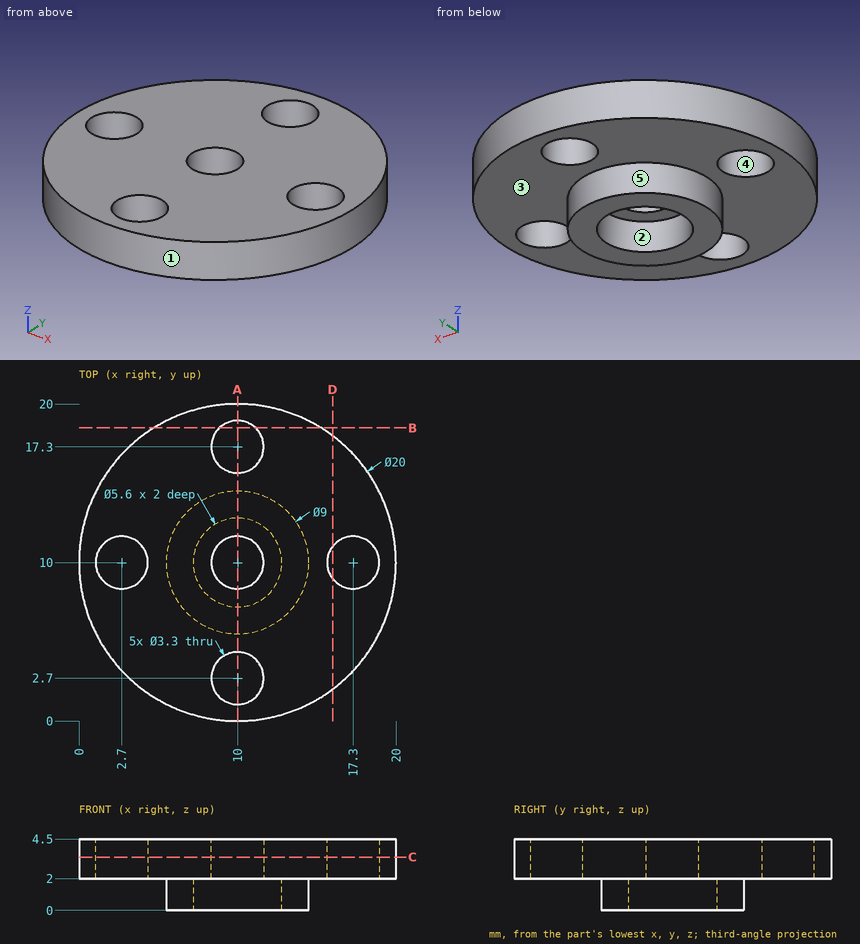
Here's the drawing with two shaded views (mm, measured from the low corner). I have some questions. A direction names the side the tool comes from. Give positions to 0.01 mm unless a question says otherwise; leave off trailing zeros. Order: outer loops, then holes, each group sorted by start corner. A loop starts at its lowest first (then second) coordinate and runs counter-clockwise, first axis right, second up. Notation, with made-up numbers: (4.5, -37) - (61.5, -37) arc R27 cw to (61.5, -1) - close; hole circle Ø9 at (58, 5). An arc over 180 degrees is marked (long way). Use a Markdown table: item, result. Add a question column.
Q1. On a 3-axis mill with a long thin cutter (end or side, diameter ignored), from which of +Z, -Z, +X, -X, +Y, -Y can I reach the whole of each face in a straight line? I mean the marked faces 4 and 5. Say none if no direction works.
Q2. If we section it at D-D on x = 16: Write out the boundary of the cut face in (y, z).
Q3. If we section it at B-B on y = 18.5: Write out the boundary of the cut face in (x, z).
Q4. If we section it at C-C on z = 3.35: Write out the boundary of the cut face in (x, y), plus the area to 3 significant figures.
Q5. If we section it at A-A on x = 10: Write out the boundary of the cut face in (y, z), plus the area to 4 significant figures.
Q6. Please list where these lines run through material, in increasing order: line 1 along Y through (x, z) = (10, 3.45); line 2 along Z through (x, y) = (7, 14.75); line 3 along X through (y, z) = (12, 1.35).
Q7. If we mould it in two halves opening along Y, with no side actions, what happens to the marked faces 1, 2 and 3? For each: released by +Y, released by -Y, zero draft, split by the parting line, or undercut.
Q8. I'm going to push flat-ended pins straight in: pin 1 (6 mm diameter, centred on x = 17.5, y = 9, fed in from -Z); pin 2 (2 mm diameter, centred on y = 13, z = 2, fed in from -X). Where does each tip first touch, or does it pass through?
Answers follow:
| question | item | result |
|---|---|---|
| 1 | face 4 | +Z, -Z |
| 1 | face 5 | -Z |
| 2 | outline | (2, 2) - (8.98, 2) - (8.98, 4.5) - (2, 4.5) - close; (11.02, 2) - (18, 2) - (18, 4.5) - (11.02, 4.5) - close |
| 3 | outline | (4.73, 2) - (8.87, 2) - (8.87, 4.5) - (4.73, 4.5) - close; (11.13, 2) - (15.27, 2) - (15.27, 4.5) - (11.13, 4.5) - close |
| 4 | outline | circle Ø20 at (10, 10); hole circle Ø3.3 at (2.7, 10); hole circle Ø3.3 at (10, 2.7); hole circle Ø3.3 at (10, 10); hole circle Ø3.3 at (10, 17.3); hole circle Ø3.3 at (17.3, 10) |
| 4 | area | 271 mm^2 |
| 5 | outline | (0, 2) - (1.05, 2) - (1.05, 4.5) - (0, 4.5) - close; (4.35, 2) - (5.5, 2) - (5.5, 0) - (7.2, 0) - (7.2, 2) - (8.35, 2) - (8.35, 4.5) - (4.35, 4.5) - close; (11.65, 2) - (12.8, 2) - (12.8, 0) - (14.5, 0) - (14.5, 2) - (15.65, 2) - (15.65, 4.5) - (11.65, 4.5) - close; (18.95, 2) - (20, 2) - (20, 4.5) - (18.95, 4.5) - close |
| 5 | area | 32.05 mm^2 |
| 6 | line 1 | y = 0 to 1.05, 4.35 to 8.35, 11.65 to 15.65, 18.95 to 20 |
| 6 | line 2 | z = 2 to 4.5 |
| 6 | line 3 | x = 5.97 to 8.04, 11.96 to 14.03 |
| 7 | face 1 | split by the parting line |
| 7 | face 2 | undercut |
| 7 | face 3 | zero draft |
| 8 | pin 1 | stops at z = 2 |
| 8 | pin 2 | stops at x = 0.2 |
